Can you work these out from the drawing? Everything is in mm from the part's minimum corner. Coordinates: 2 decimals unless noted, no trailing zeros. Order: outer loops, then holes, each group sorted by start corner. A loop starts at its lowest first (then second) coordinate and runs counter-clockwise, first axis right, second up. Notation, with made-up numbers: (22, 35.5) -> (76, 35.5) arc R17 cw to (76, 42.5) -> close; hole circle Ø6 at (64, 55.25). An arc over 180 degrees is marked (long way). Return JSON: item names as keys, results as strings. Group by question number.
1) If we section it at C-C, the plane x = 106.5: Please give me the cut outline in (y, z), then the cut area to 3 significant figures.
2) For pin 1 (0.6 mm diameter, centred on y = 0.5, z = 19, fed in from -X), with a flat end and sliding along its axis, tell me the tip position at first contact or that it passes through.
3) If we section it at A-A, the plane z = 17.5: Please give me the cut outline in (x, y), then the cut area to 3 significant figures.
4) If we section it at B-B, the plane y = 1.05: Please give me the cut outline in (x, z), then the cut area to 3 significant figures.
5) If I drill on probe 1 along X at (y, z) = (1.2, 19.5); probe 2 along Z at (x, y) = (20.5, 1.1), over which ranges is the centre line in solid material (lowest first)? Write a range as from..to.
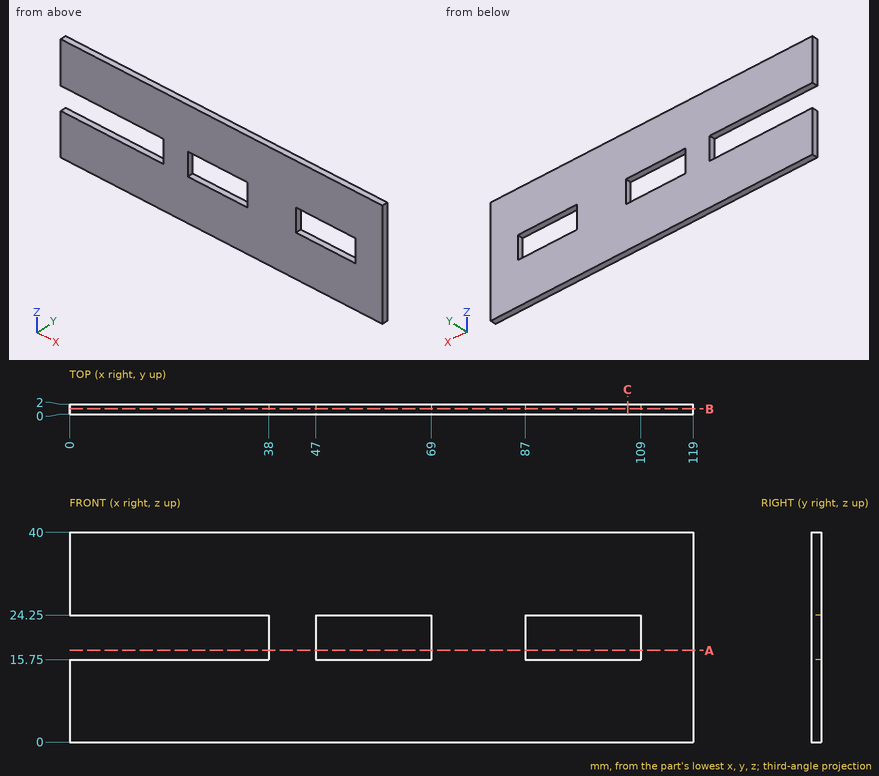
Result sheet:
{
 "1": {"outline": "(0, 0) -> (2, 0) -> (2, 15.75) -> (0, 15.75) -> close; (0, 24.25) -> (2, 24.25) -> (2, 40) -> (0, 40) -> close", "area": "63.0 mm2"},
 "2": {"pin 1": "stops at x = 38"},
 "3": {"outline": "(38, 0) -> (47, 0) -> (47, 2) -> (38, 2) -> close; (69, 0) -> (87, 0) -> (87, 2) -> (69, 2) -> close; (109, 0) -> (119, 0) -> (119, 2) -> (109, 2) -> close", "area": "74.0 mm2"},
 "4": {"outline": "(0, 0) -> (119, 0) -> (119, 40) -> (0, 40) -> (0, 24.25) -> (38, 24.25) -> (38, 15.75) -> (0, 15.75) -> close; hole (47, 15.75) -> (69, 15.75) -> (69, 24.25) -> (47, 24.25) -> close; hole (87, 15.75) -> (109, 15.75) -> (109, 24.25) -> (87, 24.25) -> close", "area": "4,060 mm2"},
 "5": {"probe 1": "x = 38..47, 69..87, 109..119", "probe 2": "z = 0..15.75, 24.25..40"}
}
